The listing builds one solid part. Answer for the finished solid, in the listing's coordinates (mm). Face numbers are marked on the shaded views. A direction names the side the tool comes from. Coordinates: 2 decimals unless noted, no trailing zeros. Loops run counter-clockwise (first coordinate to the right, second up) from the corner with the lowest first, then second, coordinate; pieces in that order, holes last. Notation, with made-up numbers: (41.5, 66.25) - (73.5, 66.25) arc R19 ccw to (73.5, 81.25) - close; hole circle Ø6 at (-36.75, 70). An arc over 180 degrees is marked (long way). Write each question's results on one line, items separated by ' | '. Start each with the question number.
(1) Given pin 1 Ø1.2 at (x, z) = (2.5, 2.5) entering from -Y; pin 2 Ø6 at (x, z) = (2, 6.5) entering from -Y; pin 3 Ø6 at (y, z) = (-8, 7.5) entering from +X; pin 4 Ø2.5 at (y, z) = (-4.5, 6.5) entering from -X, each flat-ended and moving along its own axis, determine where each tip first touches the part or whether it passes through.
(2) Find section D-D on y = 1. Determine the outline of the cut face in (x, z), then the cut area to 3 significant figures.
(3) Consider line 1 (Z direction, x = 2.5, y = 1.75); line 2 (X direction, y = -7.5, z = 6.5). Determine where each line is inside the solid, lowest interval first. Write a range as from..to.
(4) Determine the mould class of the marked faces 6, 7, 8 and 9 for opening direction X: released by +X, released by -X, zero draft, split by the parting line, or undercut.
(5) For the marked faces 1, 2, 3, 4 and 5, determine the directions among +Z, -Z, +X, -X, +Y, -Y from which every point of the face is accessible in a straight line to the end or side of a thin tool.
(6) Find section A-A on y = -6.5. Determine the outline of the cut face in (x, z), then the cut area to 3 significant figures.
(7) Find section C-C on x = 2.75. Determine the outline of the cut face in (y, z), then the cut area to 3 significant figures.
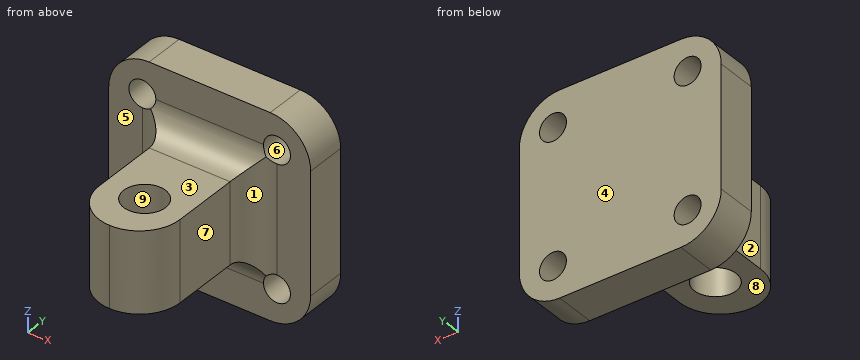
from build123d import *

# Parameters (mm, degrees)
SKETCH1_W           = 15
SKETCH1_H           = 15
BOSS_EXTRUDE1_DEPTH = 3
SKETCH3_R           = 1
CUT_EXTRUDE1_DEPTH  = 22.424285286
FILLET1_R           = 3
SKETCH4_W           = 6
SKETCH4_H           = 6
BOSS_EXTRUDE2_DEPTH = 10
SKETCH5_R           = 1.55
CUT_EXTRUDE2_DEPTH  = 21.862646045
FILLET2_R           = 3
FILLET3_R           = 2


# Some blends are built 0.0001 mm under size
with BuildPart() as part:
    # Sketch1 → Boss-Extrude1 (new body)
    with BuildSketch(Plane(origin=(0, 0, 0), x_dir=(1, 0, 0), z_dir=(0, 1, 0))):
        with Locations((7.5, -7.5)):
            Rectangle(SKETCH1_W, SKETCH1_H)
    extrude(amount=BOSS_EXTRUDE1_DEPTH)

    # Sketch3 → Cut-Extrude1 (cut, through all)
    with BuildSketch(Plane(origin=(0, 3, 0), x_dir=(1, 0, 0), z_dir=(0, 1, 0))):
        with Locations(Location((2.5, -12.5, 0), (0, 0, 270))):
            Circle(SKETCH3_R)
        with Locations(Location((12.5, -12.5, 0), (0, 0, 270))):
            Circle(SKETCH3_R)
        with Locations(Location((12.5, -2.5, 0), (0, 0, 270))):
            Circle(SKETCH3_R)
        with Locations(Location((2.5, -2.5, 0), (0, 0, 270))):
            Circle(SKETCH3_R)
    extrude(amount=-CUT_EXTRUDE1_DEPTH, mode=Mode.SUBTRACT)

    # Fillet1
    fillet1_edges = [part.edges().sort_by_distance(p)[0] for p in [
        (0, 1.5, 0),
        (15, 1.5, 0),
        (15, 1.5, 15),
        (0, 1.5, 15),
    ]]
    fillet(fillet1_edges, radius=FILLET1_R)

    # Sketch4 → Boss-Extrude2 (add)
    with BuildSketch(Plane(origin=(0, 0, 0), x_dir=(-1, 0, 0), z_dir=(0, -1, 0))):
        with Locations((-7.5, -7.5)):
            Rectangle(SKETCH4_W, SKETCH4_H)
    extrude(amount=BOSS_EXTRUDE2_DEPTH)

    # Sketch5 → Cut-Extrude2 (cut, through all)
    with BuildSketch(Plane(origin=(0, 0, 4.5), x_dir=(-1, 0, 0), z_dir=(0, 0, -1))):
        with Locations((-7.5, -6.5)):
            Circle(SKETCH5_R)
    extrude(amount=-CUT_EXTRUDE2_DEPTH, mode=Mode.SUBTRACT)

    # Fillet2
    fillet2_edges = [part.edges().sort_by_distance(p)[0] for p in [
        (10.5, -10, 7.5),
        (4.5, -10, 7.5),
    ]]
    fillet(fillet2_edges, radius=FILLET2_R - 0.0001)  # a hair under: the kernel refuses the full size

    # Fillet3
    # the kernel refuses this fillet: 2 mm, written as the material it adds along each edge
    with BuildSketch(Plane(origin=(10.5, 0, 10.5), x_dir=(0, -1, 0), z_dir=(0, 0, -1)), Plane(origin=(4.5, 0, 10.5), x_dir=(0, -1, 0), z_dir=(1, 0, 0))) as fillet3_piece_1:
        with BuildLine():
            CenterArc((FILLET3_R, -FILLET3_R), FILLET3_R, 90, 90)
            Line((0, -FILLET3_R), (0, 0))
            Line((0, 0), (FILLET3_R, 0))
        make_face()
    extrude(amount=6)
    with BuildSketch(Plane(origin=(4.5, 0, 4.5), x_dir=(-1, 0, 0), z_dir=(0, 0, 1)), Plane(origin=(10.5, 0, 4.5), x_dir=(0, 0, -1), z_dir=(-1, 0, 0))) as fillet3_piece_2:
        with BuildLine():
            CenterArc((FILLET3_R, FILLET3_R), FILLET3_R, 180, 90)
            Line((0, FILLET3_R), (0, 0))
            Line((0, 0), (FILLET3_R, 0))
        make_face()
    extrude(amount=6)
    with BuildSketch(Plane(origin=(10.5, 0, 15.5), x_dir=(0, -1, 0), z_dir=(0, 0, -1))) as fillet3_piece_3a_section:
        with BuildLine():
            CenterArc((FILLET3_R, -FILLET3_R), FILLET3_R, 90, 90)
            Line((0, -FILLET3_R), (0, 0))
            Line((0, 0), (FILLET3_R, 0))
        make_face()
    fillet3_piece_3a = extrude(amount=11, mode=Mode.PRIVATE)
    fillet3_piece_3a = split(fillet3_piece_3a, bisect_by=Plane(origin=(10.928031961, -0.460476413, 10.5), z_dir=(0, 0, 1)), keep=Keep.TOP, mode=Mode.PRIVATE)
    fillet3_piece_3a = fillet3_piece_3a & Plane(origin=(12, -0.460476413, 12), x_dir=(1, 0, 0), z_dir=(0, 1, 0)) * Cylinder(3, 30, mode=Mode.PRIVATE)
    fillet3_piece_3a = fillet3_piece_3a - Plane(origin=(12.5, -0.460476413, 12.5), x_dir=(0, 0, 1), z_dir=(0, 1, 0)) * Cylinder(1, 30, mode=Mode.PRIVATE)
    with BuildSketch(Plane(origin=(4.5, 0, 10.5), x_dir=(0, -1, 0), z_dir=(1, 0, 0))) as fillet3_piece_3b_section:
        with BuildLine():
            CenterArc((FILLET3_R, -FILLET3_R), FILLET3_R, 90, 90)
            Line((0, -FILLET3_R), (0, 0))
            Line((0, 0), (FILLET3_R, 0))
        make_face()
    fillet3_piece_3b = extrude(amount=11, mode=Mode.PRIVATE)
    fillet3_piece_3b = split(fillet3_piece_3b, bisect_by=Plane(origin=(10.5, -0.460476368, 10.928032026), z_dir=(1, 0, 0)), keep=Keep.TOP, mode=Mode.PRIVATE)
    fillet3_piece_3b = fillet3_piece_3b & Plane(origin=(12, -0.460476368, 12), x_dir=(1, 0, 0), z_dir=(0, 1, 0)) * Cylinder(3, 31, mode=Mode.PRIVATE)
    fillet3_piece_3b = fillet3_piece_3b - Plane(origin=(12.5, -0.460476368, 12.5), x_dir=(0, 0, 1), z_dir=(0, 1, 0)) * Cylinder(1, 31, mode=Mode.PRIVATE)
    fillet3_piece_3 = fillet3_piece_3a & fillet3_piece_3b
    add(fillet3_piece_3)
    with BuildSketch(Plane(origin=(10.5, 0, 10.5), x_dir=(0, -1, 0), z_dir=(0, 0, -1))) as fillet3_piece_4a_section:
        with BuildLine():
            CenterArc((FILLET3_R, -FILLET3_R), FILLET3_R, 90, 90)
            Line((0, -FILLET3_R), (0, 0))
            Line((0, 0), (FILLET3_R, 0))
        make_face()
    fillet3_piece_4a = extrude(amount=11, mode=Mode.PRIVATE)
    fillet3_piece_4a = split(fillet3_piece_4a, bisect_by=Plane(origin=(10.928032026, -0.460476368, 4.5), z_dir=(0, 0, -1)), keep=Keep.TOP, mode=Mode.PRIVATE)
    fillet3_piece_4a = fillet3_piece_4a & Plane(origin=(12, -0.460476368, 3), x_dir=(0, 0, -1), z_dir=(0, 1, 0)) * Cylinder(3, 30, mode=Mode.PRIVATE)
    fillet3_piece_4a = fillet3_piece_4a - Plane(origin=(12.5, -0.460476368, 2.5), x_dir=(0, 0, 1), z_dir=(0, 1, 0)) * Cylinder(1, 30, mode=Mode.PRIVATE)
    with BuildSketch(Plane(origin=(15.5, 0, 4.5), x_dir=(0, 0, -1), z_dir=(-1, 0, 0))) as fillet3_piece_4b_section:
        with BuildLine():
            CenterArc((FILLET3_R, FILLET3_R), FILLET3_R, 180, 90)
            Line((0, FILLET3_R), (0, 0))
            Line((0, 0), (FILLET3_R, 0))
        make_face()
    fillet3_piece_4b = extrude(amount=11, mode=Mode.PRIVATE)
    fillet3_piece_4b = split(fillet3_piece_4b, bisect_by=Plane(origin=(10.5, -0.460476818, 4.071968325), z_dir=(1, 0, 0)), keep=Keep.TOP, mode=Mode.PRIVATE)
    fillet3_piece_4b = fillet3_piece_4b & Plane(origin=(12, -0.460476818, 3), x_dir=(0, 0, -1), z_dir=(0, 1, 0)) * Cylinder(3, 30, mode=Mode.PRIVATE)
    fillet3_piece_4b = fillet3_piece_4b - Plane(origin=(12.5, -0.460476818, 2.5), x_dir=(0, 0, 1), z_dir=(0, 1, 0)) * Cylinder(1, 30, mode=Mode.PRIVATE)
    fillet3_piece_4 = fillet3_piece_4a & fillet3_piece_4b
    add(fillet3_piece_4)
    with BuildSketch(Plane(origin=(-0.5, 0, 10.5), x_dir=(0, -1, 0), z_dir=(1, 0, 0))) as fillet3_piece_5a_section:
        with BuildLine():
            CenterArc((FILLET3_R, -FILLET3_R), FILLET3_R, 90, 90)
            Line((0, -FILLET3_R), (0, 0))
            Line((0, 0), (FILLET3_R, 0))
        make_face()
    fillet3_piece_5a = extrude(amount=11, mode=Mode.PRIVATE)
    fillet3_piece_5a = split(fillet3_piece_5a, bisect_by=Plane(origin=(4.5, -0.460476374, 10.928031998), z_dir=(-1, 0, 0)), keep=Keep.TOP, mode=Mode.PRIVATE)
    fillet3_piece_5a = fillet3_piece_5a & Plane(origin=(3, -0.460476374, 12), x_dir=(-1, 0, 0), z_dir=(0, 1, 0)) * Cylinder(3, 30, mode=Mode.PRIVATE)
    fillet3_piece_5a = fillet3_piece_5a - Plane(origin=(2.5, -0.460476374, 12.5), x_dir=(0, 0, 1), z_dir=(0, 1, 0)) * Cylinder(1, 30, mode=Mode.PRIVATE)
    with BuildSketch(Plane(origin=(4.5, 0, 4.5), x_dir=(-1, 0, 0), z_dir=(0, 0, 1))) as fillet3_piece_5b_section:
        with BuildLine():
            CenterArc((FILLET3_R, FILLET3_R), FILLET3_R, 180, 90)
            Line((0, FILLET3_R), (0, 0))
            Line((0, 0), (FILLET3_R, 0))
        make_face()
    fillet3_piece_5b = extrude(amount=11, mode=Mode.PRIVATE)
    fillet3_piece_5b = split(fillet3_piece_5b, bisect_by=Plane(origin=(4.071967841, -0.460476686, 10.5), z_dir=(0, 0, 1)), keep=Keep.TOP, mode=Mode.PRIVATE)
    fillet3_piece_5b = fillet3_piece_5b & Plane(origin=(3, -0.460476686, 12), x_dir=(-1, 0, 0), z_dir=(0, 1, 0)) * Cylinder(3, 30, mode=Mode.PRIVATE)
    fillet3_piece_5b = fillet3_piece_5b - Plane(origin=(2.5, -0.460476686, 12.5), x_dir=(0, 0, 1), z_dir=(0, 1, 0)) * Cylinder(1, 30, mode=Mode.PRIVATE)
    fillet3_piece_5 = fillet3_piece_5a & fillet3_piece_5b
    add(fillet3_piece_5)
    with BuildSketch(Plane(origin=(4.5, 0, -0.5), x_dir=(-1, 0, 0), z_dir=(0, 0, 1))) as fillet3_piece_6a_section:
        with BuildLine():
            CenterArc((FILLET3_R, FILLET3_R), FILLET3_R, 180, 90)
            Line((0, FILLET3_R), (0, 0))
            Line((0, 0), (FILLET3_R, 0))
        make_face()
    fillet3_piece_6a = extrude(amount=11, mode=Mode.PRIVATE)
    fillet3_piece_6a = fillet3_piece_6a & Plane(origin=(3, -0.460476683, 3), x_dir=(0, 0, -1), z_dir=(0, 1, 0)) * Cylinder(3, 30, mode=Mode.PRIVATE)
    fillet3_piece_6a = fillet3_piece_6a - Plane(origin=(2.5, -0.460476683, 2.5), x_dir=(0, 0, 1), z_dir=(0, 1, 0)) * Cylinder(1, 30, mode=Mode.PRIVATE)
    fillet3_piece_6a = split(fillet3_piece_6a, bisect_by=Plane(origin=(4.071967813, -0.460476683, 4.5), z_dir=(0, 0, -1)), keep=Keep.TOP, mode=Mode.PRIVATE)
    with BuildSketch(Plane(origin=(10.5, 0, 4.5), x_dir=(0, 0, -1), z_dir=(-1, 0, 0))) as fillet3_piece_6b_section:
        with BuildLine():
            CenterArc((FILLET3_R, FILLET3_R), FILLET3_R, 180, 90)
            Line((0, FILLET3_R), (0, 0))
            Line((0, 0), (FILLET3_R, 0))
        make_face()
    fillet3_piece_6b = extrude(amount=11, mode=Mode.PRIVATE)
    fillet3_piece_6b = fillet3_piece_6b & Plane(origin=(3, -0.460476796, 3), x_dir=(0, 0, -1), z_dir=(0, 1, 0)) * Cylinder(3, 30, mode=Mode.PRIVATE)
    fillet3_piece_6b = fillet3_piece_6b - Plane(origin=(2.5, -0.460476796, 2.5), x_dir=(0, 0, 1), z_dir=(0, 1, 0)) * Cylinder(1, 30, mode=Mode.PRIVATE)
    fillet3_piece_6b = split(fillet3_piece_6b, bisect_by=Plane(origin=(4.5, -0.460476796, 4.071968238), z_dir=(-1, 0, 0)), keep=Keep.TOP, mode=Mode.PRIVATE)
    fillet3_piece_6 = fillet3_piece_6a & fillet3_piece_6b
    add(fillet3_piece_6)


solid = part.part
Values:
1) pin 1: passes through | pin 2: stops at y = -8.66 | pin 3: stops at x = 10.5 | pin 4: stops at x = 4.5
2) outline: (0, 3) arc R3 ccw to (3, 0) - (12, 0) arc R3 ccw to (15, 3) - (15, 12) arc R3 ccw to (12, 15) - (3, 15) arc R3 ccw to (0, 12) - close; hole circle Ø2 at (2.5, 2.5); hole circle Ø2 at (2.5, 12.5); hole circle Ø2 at (12.5, 2.5); hole circle Ø2 at (12.5, 12.5) | area: 205 mm²
3) line 1: z = 0.04..1.5, 3.5..11.5, 13.5..14.96 | line 2: x = 4.54..6.32, 8.68..10.46
4) face 6: undercut | face 7: released by +X | face 8: zero draft | face 9: undercut
5) face 1: +Z, -Z, +X, -Y | face 2: +Z, -Z, -X, -Y | face 3: +Z, +X, -X, -Y | face 4: +Z, -Z, +X, -X, +Y | face 5: -Y
6) outline: (4.5, 4.5) - (5.95, 4.5) - (5.95, 10.5) - (4.5, 10.5) - close; (9.05, 4.5) - (10.5, 4.5) - (10.5, 10.5) - (9.05, 10.5) - close | area: 17.4 mm²
7) outline: (-0.02, 3.47) - (3, 3.47) - (3, 11.53) - (-0.02, 11.53) - close; (0, 0.01) - (3, 0.01) - (3, 1.53) - (0, 1.53) - close; (0, 13.47) - (3, 13.47) - (3, 14.99) - (0, 14.99) - close | area: 33.4 mm²
